```python
from build123d import *

# Parameters (mm, degrees)
SKETCH1_W           = 19.05
SKETCH1_H           = 19.05
BOSS_EXTRUDE1_DEPTH = 177.8
BOSS_EXTRUDE2_DEPTH = 7.62
SKETCH3_R           = 2.54
CUT_EXTRUDE1_DEPTH  = 7.62
SKETCH4_R           = 4.445
CUT_EXTRUDE2_DEPTH  = 19.05
SKETCH5_R           = 3.175
SKETCH5_R_2         = 2.54
CUT_EXTRUDE3_DEPTH  = 38.1
SKETCH6_W           = 19.05
SKETCH6_H           = 12.7
BOSS_EXTRUDE3_DEPTH = 25.4


with BuildPart() as part:
    # Sketch1 → Boss-Extrude1 (new body)
    with BuildSketch(Plane(origin=(0, 0, 0), x_dir=(1, 0, 0), z_dir=(0, 1, 0))):
        with Locations((9.525, 9.525)):
            Rectangle(SKETCH1_W, SKETCH1_H)
    extrude(amount=BOSS_EXTRUDE1_DEPTH)

    # Sketch2 → Boss-Extrude2 (add)
    with BuildSketch(Plane.XZ):
        with BuildLine():
            ThreePointArc((34.925, -12.7), (2.950996254, 11.834515988), (-12.472045256, -25.4))
            Line((-12.472045256, -25.4), (31.522045256, -25.4))
            ThreePointArc((31.522045256, -25.4), (34.059515988, -19.274003746), (34.925, -12.7))
        make_face()
    extrude(amount=BOSS_EXTRUDE2_DEPTH)

    # Sketch3 → Cut-Extrude1 (cut)
    with BuildSketch(Plane(origin=(0, 0, 0), x_dir=(1, 0, 0), z_dir=(0, 1, 0))):
        with Locations((-6.35, 9.525)):
            Circle(SKETCH3_R)
        with Locations((25.4, 9.525)):
            Circle(SKETCH3_R)
        with Locations((9.525, -6.35)):
            Circle(SKETCH3_R)
    extrude(amount=-CUT_EXTRUDE1_DEPTH, mode=Mode.SUBTRACT)

    # Sketch4 → Cut-Extrude2 (cut)
    with BuildSketch(Plane(origin=(0, 0, -19.05), x_dir=(-1, 0, 0), z_dir=(0, 0, -1))):
        with Locations((-9.525, 165.1)):
            Circle(SKETCH4_R)
    extrude(amount=-CUT_EXTRUDE2_DEPTH, mode=Mode.SUBTRACT)

    # Sketch5 → Cut-Extrude3 (cut)
    with BuildSketch(Plane(origin=(0, 0, -19.05), x_dir=(-1, 0, 0), z_dir=(0, 0, -1))):
        with Locations((-9.525, 134.62)):
            Circle(SKETCH5_R)
        with Locations((-9.525, 113.03)):
            Circle(SKETCH5_R_2)
    extrude(amount=-CUT_EXTRUDE3_DEPTH, mode=Mode.SUBTRACT)

    # Sketch6 → Boss-Extrude3 (add)
    with BuildSketch(Plane(origin=(0, 0, -19.05), x_dir=(-1, 0, 0), z_dir=(0, 0, -1))):
        with Locations((-9.525, 100.33)):
            Rectangle(SKETCH6_W, SKETCH6_H)
    extrude(amount=BOSS_EXTRUDE3_DEPTH)


solid = part.part
```
Source: CAD feature listing. Evaluate the final solid. Frame: model axes, mm. A direction names the side the tool comes from. Round coordinates to 2 decimals unless told otherwise and drop trailing zeros. Loops run counter-clockwise (first coordinate to the right, second up) from the corner with the lowest first, then second, coordinate; pieces in that order, holes last. Notation, with made-up numbers: M 69.5,23 L 85.5,23 A29 cw 85.5,55 Z; hole C 32,79 d8. An arc over 180 degrees is marked long. Put each result on its own line as item: value.
(1) First-contact query: pin 1 (2 mm diameter, centred on x = -9, z = 1.5, fed in from +Y); pin 2 (6 mm diameter, centred on y = 77, z = -22, fed in from +X); pin 3 (9.5 mm diameter, centred on x = 5, z = -30.5, fed in from +Y). Flat tips, straight axial feed; report the tip coordinate or a pass-through.
Solutions:
pin 1: y = 0
pin 2: x = 19.05
pin 3: y = 106.68
(2) Section A-A, the plane x = 26. Return loops of the section in (y, z), and give its area (3 significant figures).
Solutions:
outline: M -7.62,-25.4 L 0,-25.4 L 0,-11.99 L -7.62,-11.99 Z; M -7.62,-7.06 L 0,-7.06 L 0,6.63 L -7.62,6.63 Z
area: 206 mm²
(3) Section C-C, the plane y = 158. Return loops of the section in (x, z), and give its area (3 significant figures).
Solutions:
outline: M 0,-19.05 L 19.05,-19.05 L 19.05,0 L 0,0 Z
area: 363 mm²
(4) Pull-direction query (X, two-part tool) for faces 6 (the face through (9, 0, 2)), 7 (the face through (9.938, 137.768, -9.658)), 8 (the face through (19.05, 88, -7)); classes: released by +X, released by -X, zero draft, split by the parting line, or undercut.
Solutions:
face 6: zero draft
face 7: undercut
face 8: released by +X
(5) Access query for faces 1 (the face through (9, 88, 0)), 2 (the face through (0, 88, -7)), 3 (the face through (9, -4, -25.4)), 4 (the face through (9, 46, -19.05)), 5 (the face through (9, 142, -19.05)). Directions: +Z, -Z, +X, -X, +Y, -Y. A direction counts if a zero-diameter tool reaches every point of the face in a straight line with its end or side. Return the directions, or none.
Solutions:
face 1: +Z, +X, -X, +Y
face 2: +Z, -Z, -X, +Y
face 3: -Z, +X, -X, -Y
face 4: -Z, +X, -X
face 5: -Z, +X, -X, +Y
(6) Ray query, line 1 (Y direction, x = 19, z = -32.5); line 2 (Z direction, x = 5.5, y = 91); line 3 (Y direction, x = 20.5, z = 2.5). Return the intervals inside material, ascending. Write a range as [from, to].
Solutions:
line 1: [93.98, 106.68]
line 2: [-19.05, 0]
line 3: [-7.62, 0]
(7) Section B-B, the plane z = -2. Return loops of the section in (x, y) (3 decimals).
Solutions:
outline: M -13.511,-7.62 L 32.561,-7.62 L 32.561,0 L 19.05,0 L 19.05,177.8 L 0,177.8 L 0,0 L -13.511,0 Z; hole C 9.525,165.1 d8.89; hole C 9.525,134.62 d6.35; hole C 9.525,113.03 d5.08
(8) Section D-D, the plane z = -38.5. Return loops of the section in (x, y), and give its area (3 significant figures).
Solutions:
outline: M 0,93.98 L 19.05,93.98 L 19.05,106.68 L 0,106.68 Z
area: 242 mm²
